For this review, take the finished solid that the model builds, in its own axes (mm). A direction names the side the tool comes from. Round coordinates to 2 decimals unless told otherwise and drop trailing zeros. Write each loop counter-clockwise with the first axis right and the second up, starting at its lowest first coordinate (ties: lowest second). Pieces come first, ordered by that corner, then holes.
from build123d import *

# Parameters (mm, degrees)
SKETCH1_W                    = 370
SKETCH1_H                    = 60
BASE_FLANGE1_DEPTH           = 6
EDGE_FLANGE1_STRIP_W         = 36
EDGE_FLANGE1_STRIP_H         = 6
EDGE_FLANGE1_STRIP_CUT_DEPTH = 60
EDGE_FLANGE1_DEPTH           = 60
EDGE_FLANGE2_STRIP_W         = 36
EDGE_FLANGE2_STRIP_H         = 6
EDGE_FLANGE2_STRIP_CUT_DEPTH = 60
EDGE_FLANGE2_DEPTH           = 60
EDGE_FLANGE3_STRIP_W         = 36
EDGE_FLANGE3_STRIP_H         = 6
EDGE_FLANGE3_STRIP_CUT_DEPTH = 60
EDGE_FLANGE3_DEPTH           = 60
EDGE_FLANGE4_STRIP_W         = 36
EDGE_FLANGE4_STRIP_H         = 6
EDGE_FLANGE4_STRIP_CUT_DEPTH = 60
EDGE_FLANGE4_DEPTH           = 60
SKETCH18_R                   = 15
SKETCH18_R_2                 = 5
SKETCH18_R_3                 = 3.25
CUT_EXTRUDE1_DEPTH           = 65
CUT_EXTRUDE2_DEPTH           = 65
SKETCH23_R                   = 2.5
CUT_EXTRUDE3_DEPTH           = 6
FILLET1_R                    = 5


# Sheet-metal steps are written as plain solids
with BuildPart() as part:
    # Sketch1 → Base-Flange1 (new body)
    with BuildSketch(Plane.XY):
        Rectangle(SKETCH1_W, SKETCH1_H)
    extrude(amount=-BASE_FLANGE1_DEPTH)

    # Edge-Flange1 strip (across the edge) → Edge-Flange1 strip cut (cut)
    with BuildSketch(Plane(origin=(185, -30, 0), x_dir=(-1, 0, 0), z_dir=(0, 1, 0))):
        with Locations((-6, -3)):
            Rectangle(EDGE_FLANGE1_STRIP_W, EDGE_FLANGE1_STRIP_H)
    extrude(amount=EDGE_FLANGE1_STRIP_CUT_DEPTH, mode=Mode.SUBTRACT)

    # Edge-Flange1 section (across the edge) → Edge-Flange1 (add)
    with BuildSketch(Plane(origin=(185, -30, 0), x_dir=(-1, 0, 0), z_dir=(0, 1, 0))):
        with BuildLine():
            Line((0, 6), (0, 294))
            Line((0, 294), (6, 294))
            Line((6, 294), (6, 6))
            ThreePointArc((6, 6), (7.757359313, 1.757359313), (12, 0))
            Line((12, 0), (12, -6))
            ThreePointArc((12, -6), (3.514718626, -2.485281374), (0, 6))
        make_face()
    extrude(amount=EDGE_FLANGE1_DEPTH)

    # Edge-Flange2 strip (across the edge) → Edge-Flange2 strip cut (cut)
    with BuildSketch(Plane(origin=(-185, 30, 0), x_dir=(1, 0, 0), z_dir=(0, -1, 0))):
        with Locations((-6, -3)):
            Rectangle(EDGE_FLANGE2_STRIP_W, EDGE_FLANGE2_STRIP_H)
    extrude(amount=EDGE_FLANGE2_STRIP_CUT_DEPTH, mode=Mode.SUBTRACT)

    # Edge-Flange2 section (across the edge) → Edge-Flange2 (add)
    with BuildSketch(Plane(origin=(-185, 30, 0), x_dir=(1, 0, 0), z_dir=(0, -1, 0))):
        with BuildLine():
            Line((0, 6), (0, 294))
            Line((0, 294), (6, 294))
            Line((6, 294), (6, 6))
            ThreePointArc((6, 6), (7.757359313, 1.757359313), (12, 0))
            Line((12, 0), (12, -6))
            ThreePointArc((12, -6), (3.514718626, -2.485281374), (0, 6))
        make_face()
    extrude(amount=EDGE_FLANGE2_DEPTH)

    # Edge-Flange3 strip (across the edge) → Edge-Flange3 strip cut (cut)
    with BuildSketch(Plane(origin=(185, 30, 294), x_dir=(0, 0, -1), z_dir=(0, -1, 0))):
        with Locations((-6, -3)):
            Rectangle(EDGE_FLANGE3_STRIP_W, EDGE_FLANGE3_STRIP_H)
    extrude(amount=EDGE_FLANGE3_STRIP_CUT_DEPTH, mode=Mode.SUBTRACT)

    # Edge-Flange3 section (across the edge) → Edge-Flange3 (add)
    with BuildSketch(Plane(origin=(185, 30, 294), x_dir=(0, 0, -1), z_dir=(0, -1, 0))):
        with BuildLine():
            Line((0, 6), (0, 44))
            Line((0, 44), (6, 44))
            Line((6, 44), (6, 6))
            ThreePointArc((6, 6), (7.757359313, 1.757359313), (12, 0))
            Line((12, 0), (12, -6))
            ThreePointArc((12, -6), (3.514718626, -2.485281374), (0, 6))
        make_face()
    extrude(amount=EDGE_FLANGE3_DEPTH)

    # Edge-Flange4 strip (across the edge) → Edge-Flange4 strip cut (cut)
    with BuildSketch(Plane(origin=(-185, -30, 294), x_dir=(0, 0, -1), z_dir=(0, 1, 0))):
        with Locations((-6, -3)):
            Rectangle(EDGE_FLANGE4_STRIP_W, EDGE_FLANGE4_STRIP_H)
    extrude(amount=EDGE_FLANGE4_STRIP_CUT_DEPTH, mode=Mode.SUBTRACT)

    # Edge-Flange4 section (across the edge) → Edge-Flange4 (add)
    with BuildSketch(Plane(origin=(-185, -30, 294), x_dir=(0, 0, -1), z_dir=(0, 1, 0))):
        with BuildLine():
            Line((0, 6), (0, 44))
            Line((0, 44), (6, 44))
            Line((6, 44), (6, 6))
            ThreePointArc((6, 6), (7.757359313, 1.757359313), (12, 0))
            Line((12, 0), (12, -6))
            ThreePointArc((12, -6), (3.514718626, -2.485281374), (0, 6))
        make_face()
    extrude(amount=EDGE_FLANGE4_DEPTH)

    # Sketch18 → Cut-Extrude1 (cut)
    with BuildSketch(Plane(origin=(0, 0, -6), x_dir=(-1, 0, 0), z_dir=(0, 0, -1))):
        Circle(SKETCH18_R)
        with Locations((-100, 0)):
            Circle(SKETCH18_R_2)
        with Locations((100, 0)):
            Circle(SKETCH18_R_2)
        with Locations((-16.5, 16.5)):
            Circle(SKETCH18_R_3)
        with Locations((16.5, 16.5)):
            Circle(SKETCH18_R_3)
        with Locations((16.5, -16.5)):
            Circle(SKETCH18_R_3)
        with Locations((-16.5, -16.5)):
            Circle(SKETCH18_R_3)
    extrude(amount=-CUT_EXTRUDE1_DEPTH, mode=Mode.SUBTRACT)

    # Sketch22 → Cut-Extrude2 (cut)
    with BuildSketch(Plane(origin=(0, 0, 288), x_dir=(-1, 0, 0), z_dir=(0, 0, -1))):
        with BuildLine():
            Line((-204, 16), (-214, 16))
            ThreePointArc((-214, 16), (-218, 20), (-214, 24))
            Line((-214, 24), (-204, 24))
            ThreePointArc((-204, 24), (-200, 20), (-204, 16))
        make_face()
        with BuildLine():
            Line((-204, -16), (-214, -16))
            ThreePointArc((-214, -16), (-218, -20), (-214, -24))
            Line((-214, -24), (-204, -24))
            ThreePointArc((-204, -24), (-200, -20), (-204, -16))
        make_face()
        with BuildLine():
            Line((204, 16), (214, 16))
            ThreePointArc((214, 16), (218, 20), (214, 24))
            Line((214, 24), (204, 24))
            ThreePointArc((204, 24), (200, 20), (204, 16))
        make_face()
        with BuildLine():
            Line((204, -16), (214, -16))
            ThreePointArc((214, -16), (218, -20), (214, -24))
            Line((214, -24), (204, -24))
            ThreePointArc((204, -24), (200, -20), (204, -16))
        make_face()
    extrude(amount=-CUT_EXTRUDE2_DEPTH, mode=Mode.SUBTRACT)

    # Sketch23 → Cut-Extrude3 (cut)
    with BuildSketch(Plane(origin=(0, 0, -6), x_dir=(-1, 0, 0), z_dir=(0, 0, -1))):
        with Locations((115.875233888, 0.006238306)):
            Circle(SKETCH23_R)
        with Locations((83.875233888, 0.006238306)):
            Circle(SKETCH23_R)
        with Locations((-115.875233888, 0.006238306)):
            Circle(SKETCH23_R)
        with Locations((-83.875233888, 0.006238306)):
            Circle(SKETCH23_R)
    extrude(amount=-CUT_EXTRUDE3_DEPTH, mode=Mode.SUBTRACT)

    # Fillet1
    fillet1_edges = [part.edges().sort_by_distance(p)[0] for p in [
        (229, 30, 291),
        (229, -30, 291),
        (-229, -30, 291),
        (-229, 30, 291),
    ]]
    fillet(fillet1_edges, radius=FILLET1_R)


solid = part.part
(1) We need section C-C, the plane x = -72.5. Give the boundary of the cut face in (y, z), and give its area (3 significant figures).
Geometry check:
outline: (-30, -6) - (30, -6) - (30, 0) - (-30, 0) - close
area: 360 mm2
(2) For faces 1 (the face through (-2, -20, -6)), 2 (the face through (-210, 0, 288)), 3 (the face through (185, 0, 142)), 4 (the face through (-179, 0, 146)), 5 (the face through (95.381, -1.915, -3.042)), list the 3-axis set-ups (+Z, -Z, +X, -X, +Y, -Y) from which the entire face can be reached by the end or side of a thin tool; tool diameter is ignored.
Geometry check:
face 1: -Z, +X, -X, +Y, -Y
face 2: -Z, -X, +Y, -Y
face 3: -Z, +X, +Y, -Y
face 4: +Z, +Y, -Y
face 5: +Z, -Z
(3) We need section A-A, the plane x = 0. Give the boundary of the cut face in (y, z).
Geometry check:
outline: (-30, -6) - (-15, -6) - (-15, 0) - (-30, 0) - close; (15, -6) - (30, -6) - (30, 0) - (15, 0) - close
(4) For pin 1 Ø10.5 at (x, y) = (16.5, -16.5) entering from -Z; pin 2 Ø4 at (x, y) = (16.5, 16.5) entering from +Z; pin 3 Ø12 at (y, z) = (2, 31.5) entering from +X; pin 4 Ø19 at (x, y) = (-204.5, -9.5) entering from -Z, all flat-tipped, find the tip position at first contact; note any pin that passes through.
Geometry check:
pin 1: stops at z = -6
pin 2: passes through
pin 3: stops at x = 185
pin 4: stops at z = 288
(5) We need section B-B, the plane z = 81.5. Give the boundary of the cut face in (x, y), and give its area (3 significant figures).
Geometry check:
outline: (-185, -30) - (-179, -30) - (-179, 30) - (-185, 30) - close; (179, -30) - (185, -30) - (185, 30) - (179, 30) - close
area: 720 mm2
(6) For line 1 along Y through (x, z) = (16.5, -2.6); line 2 along Y through (x, z) = (0, -1); line 3 along X through (y, z) = (15.5, 172.5), list the stretches that pass through material, from the lowest coordinate up.
Geometry check:
line 1: y = -30 to -19.75, -13.25 to 13.25, 19.75 to 30
line 2: y = -30 to -15, 15 to 30
line 3: x = -185 to -179, 179 to 185
